CAD build for the part. Positions are in the model's coordinates, mm. A direction names the side the tool comes from. Round coordinates to 2 decimals unless told otherwise and drop trailing zeros. Write each loop counter-clockwise with the first axis right and the second up, starting at its lowest first coordinate (ties: lowest second). Pieces come first, ordered by that corner, then holes. Notation, with made-up numbers: (30.25, 4.5) - (75.25, 4.5) arc R12 cw to (75.25, 18.5) - close; hole circle Ø6 at (32.25, 32.25). An arc over 180 degrees is marked (long way). Use one line per item in the form item = value. Start each with the question number.
Item 1: Band-saw the part on A-A, the plane z = -34. List the corners of the cut face in (x, y), and give its area (3 significant figures).
Item 2: Pull direction Z, two halves, no side cores. Call faces 4 (the flat face through (-5, -3, -30.162)), 5 (the flat face through (-21, -3, -23.019)), 6 (the flat face through (52, -3, -34.925)), 7 (the flat face through (-1, -6.35, -27)): +Z half, -Z half, draft (parallel to the pull), parting line (faces both ways), or undercut.
Item 3: Drill centre lines: L1, parallel to X at y = -1.5, z = -34.5; L2, parallel to X at y = -2.75, z = -34; L3, parallel to Z at x = -41, y = -5.5. Where is each one in solid material? Low to high.
Item 4: Band-saw the part on D-D, the plane x = 43. List the corners of the cut face in (y, z), and give its area (3 significant figures).
Item 5: Band-saw the part on B-B, the plane y = -2.25. Give the number of separate pieces and of enclosed holes in the cut face, and give its area (3 significant figures).
Item 6: Band-saw the part on C-C, the plane z = -42.25. List the corners of the cut face in (x, y), and give its area (3 significant figures).
Item 7: Pin check, flat tips, straight feed: pin 1 (1.5 mm diameter, centred on y = -1, z = -39, fed in from +X); pin 2 (10 mm diameter, centred on x = 9, z = -40.5, fed in from -Y); pin 3 (1.7 mm diameter, centred on y = -3, z = -26.5, fed in from -X); pin 4 (2 mm diameter, centred on y = -3.5, z = -27.5, fed in from +X). Stop position of each tip, or through.
Item 8: Tool access for faces 1 (the flat face through (14.6, -3.13, -24.03)), 2 (the flat face through (-52, -3, -34.925)), 3 (the flat face through (47.644, -3, -33)): list every direction of +Z, -Z, +X, -X, +Y, -Y with a clear straight run to the whole face (end or side of a thin tool).
from build123d import *

# Parameters (mm, degrees)
F0_W     = 6.35
F0_H     = 9.525
F0_W_2   = 1.5875
F0_H_2   = 3.96875
F0_H_3   = 3.175
F1_DEPTH = 6.35


# Not quite as in the source:
# - a length typed as a fraction of an inch, garbled in the dataset ("3 / 203.2 mm" for 3/8 in), is restored


with BuildPart() as f1:
    # F0 (on Front) → F1 (new body)
    with BuildSketch(Plane.XZ):
        Polygon((52.4060167908, -29.36875), (55.5810167908, -23.8125), (49.2310167908, -23.8125), (49.2310167908, -20.6375), (-49.1939832092, -20.6375), (-49.1939832092, -23.8125), (-55.5439832092, -23.8125), (-52.3689832092, -29.36875), (-55.5439832092, -34.925), (-47.6064832092, -34.925), (-47.6064832092, -31.75), (-3.1564832092, -31.75), (3.1935167908, -31.75), (47.6435167908, -31.75), (47.6435167908, -34.925), (55.5810167908, -34.925), align=None)
        with BuildLine():
            Line((-36.909375, -22.225), (36.909375, -22.225))
            Line((36.909375, -22.225), (36.909375, -30.1625))
            Line((36.909375, -30.1625), (34.7265625, -30.1625))
            Line((34.7265625, -30.1625), (31.5515625, -30.1625))
            Line((31.5515625, -30.1625), (28.3765625, -30.1625))
            Line((28.3765625, -30.1625), (27.1859375, -30.1625))
            Line((27.1859375, -30.1625), (20.8359375, -30.1625))
            Line((20.8359375, -30.1625), (19.6453125, -30.1625))
            Line((19.6453125, -30.1625), (17.2640625, -30.1625))
            Line((17.2640625, -30.1625), (13.6921875, -30.1625))
            Line((13.6921875, -30.1625), (11.3109375, -30.1625))
            Line((11.3109375, -30.1625), (10.1203125, -30.1625))
            Line((10.1203125, -30.1625), (7.7390625, -30.1625))
            Line((7.7390625, -30.1625), (6.1515625, -30.1625))
            Line((6.1515625, -30.1625), (3.7703125, -30.1625))
            Line((3.7703125, -30.1625), (2.5796875, -30.1625))
            Line((2.5796875, -30.1625), (0.1984375, -30.1625))
            Line((0.1984375, -30.1625), (-1.3890625, -30.1625))
            Line((-1.3890625, -30.1625), (-3.7703125, -30.1625))
            Line((-3.7703125, -30.1625), (-4.9609375, -30.1625))
            Line((-4.9609375, -30.1625), (-6.8241157772, -30.1625))
            add(Edge.make_bspline(
                [(-8.1359375, -30.1873046875), (-7.6862010464, -30.1873046875), (-7.2364645928, -30.1795465798), (-6.8241157772, -30.1625)],
                knots=[0.5, 0.5, 0.5, 0.5, 0.5965188889, 0.5965188889, 0.5965188889, 0.5965188889], degree=3))
            add(Edge.make_bspline(
                [(-9.4477592243, -30.1625), (-9.0354104083, -30.1795465799), (-8.5856739541, -30.1873046875), (-8.1359375, -30.1873046875)],
                knots=[0.403481111, 0.403481111, 0.403481111, 0.403481111, 0.5, 0.5, 0.5, 0.5], degree=3))
            Line((-9.4477592243, -30.1625), (-11.3109375, -30.1625))
            Line((-11.3109375, -30.1625), (-12.5015625, -30.1625))
            Line((-12.5015625, -30.1625), (-14.8828125, -30.1625))
            Line((-14.8828125, -30.1625), (-16.4703125, -30.1625))
            Line((-16.4703125, -30.1625), (-18.8515625, -30.1625))
            Line((-18.8515625, -30.1625), (-20.0421875, -30.1625))
            Line((-20.0421875, -30.1625), (-22.4234375, -30.1625))
            Line((-22.4234375, -30.1625), (-24.8046875, -30.1625))
            Line((-24.8046875, -30.1625), (-27.1859375, -30.1625))
            Line((-27.1859375, -30.1625), (-28.3765625, -30.1625))
            Line((-28.3765625, -30.1625), (-30.8380988479, -30.1625))
            add(Edge.make_bspline(
                [(-31.5515625, -30.1873046875), (-31.3115619086, -30.1873046875), (-31.0715613172, -30.1779187981), (-30.8380988479, -30.1625)],
                knots=[0.5, 0.5, 0.5, 0.5, 0.5625917967, 0.5625917967, 0.5625917967, 0.5625917967], degree=3))
            add(Edge.make_bspline(
                [(-32.2650261503, -30.1625), (-32.0315636815, -30.177918798), (-31.7915630907, -30.1873046875), (-31.5515625, -30.1873046875)],
                knots=[0.4374082034, 0.4374082034, 0.4374082034, 0.4374082034, 0.5, 0.5, 0.5, 0.5], degree=3))
            Line((-32.2650261503, -30.1625), (-34.7265625, -30.1625))
            Line((-34.7265625, -30.1625), (-36.909375, -30.1625))
            Line((-36.909375, -30.1625), (-36.909375, -22.225))
        make_face(mode=Mode.SUBTRACT)
        with Locations((0.0185167908, -39.6875)):
            Rectangle(F0_W, F0_H)
        Polygon((17.2640625, -30.1625), (19.6453125, -30.1625), (19.6453125, -23.01875), (17.2640625, -23.01875), (15.478125, -25.0092855764), (13.6921875, -23.01875), (11.3109375, -23.01875), (11.3109375, -30.1625), (13.6921875, -30.1625), (13.6921875, -26.5844644236), (15.478125, -28.575), (17.2640625, -26.5844644236), align=None)
        with BuildLine():
            Line((28.3765625, -30.1625), (31.5515625, -30.1625))
            add(Edge.make_bspline(
                [(31.5515625, -30.1625), (32.7421875004, -30.1591077376), (34.5123349703, -30.1090597393), (34.7058178423, -29.8567694785), (34.7265625, -29.765625)],
                knots=[0, 0, 0, 0, 0.5486856078, 0.7169739211, 0.7169739211, 0.7169739211, 0.7169739211], degree=3))
            Line((34.7265625, -29.765625), (34.7265625, -28.971875))
            Line((34.7265625, -28.971875), (34.7265625, -24.209375))
            add(Edge.make_bspline(
                [(32.338456939, -23.01875), (33.0698998056, -23.0207151841), (33.9016308923, -23.0447678149), (34.6240389102, -23.3694667004), (34.7265625, -23.8125000002), (34.7265625, -24.209375)],
                knots=[0.1152880959, 0.1152880959, 0.1152880959, 0.1152880959, 0.4729542068, 0.722889892, 1, 1, 1, 1], degree=3))
            Line((32.338456939, -23.01875), (31.5515625, -23.01875))
            Line((31.5515625, -23.01875), (28.3765625, -23.01875))
            Line((28.3765625, -23.01875), (28.3765625, -30.1625))
        make_face()
        with Locations((31.5515625, -26.590625)):
            Rectangle(F0_W_2, F0_H_2, mode=Mode.SUBTRACT)
        Polygon((-27.1859375, -23.01875), (-27.1859375, -30.1625), (-24.8046875, -30.1625), (-24.8046875, -26.9875), (-22.4234375, -30.1625), (-20.0421875, -30.1625), (-20.0421875, -23.01875), (-22.4234375, -23.01875), (-22.4234375, -26.19375), (-24.8046875, -23.01875), align=None)
        Polygon((0.1984375, -30.1625), (2.5796875, -30.1625), (2.5796875, -23.01875), (0.1984375, -23.01875), (0.1984375, -25.4), (-1.3890625, -25.4), (-1.3890625, -23.01875), (-3.7703125, -23.01875), (-3.7703125, -30.1625), (-1.3890625, -30.1625), (-1.3890625, -27.78125), (0.1984375, -27.78125), align=None)
        with BuildLine():
            add(Edge.make_bspline(
                [(-34.7265625, -28.971875), (-34.7265625, -29.3687499998), (-34.6194398399, -29.8515743848), (-33.9447907089, -29.9651114553), (-32.920864157, -30.119185827), (-32.2650261503, -30.1625)],
                knots=[0, 0, 0, 0, 0.139450599, 0.2615766049, 0.4374082034, 0.4374082034, 0.4374082034, 0.4374082034], degree=3))
            Line((-32.2650261503, -30.1625), (-31.5515625, -30.1625))
            Line((-31.5515625, -30.1625), (-30.8380988479, -30.1625))
            add(Edge.make_bspline(
                [(-30.8380988479, -30.1625), (-30.1822608419, -30.119185827), (-29.1583342909, -29.9651114555), (-28.4836851601, -29.851574384), (-28.3765625, -29.3687500019), (-28.3765625, -28.971875)],
                knots=[0.5625917967, 0.5625917967, 0.5625917967, 0.5625917967, 0.7384233951, 0.860549401, 1, 1, 1, 1], degree=3))
            Line((-28.3765625, -28.971875), (-28.3765625, -23.01875))
            Line((-28.3765625, -23.01875), (-30.7578125, -23.01875))
            Line((-30.7578125, -23.01875), (-30.7578125, -28.575))
            Line((-30.7578125, -28.575), (-32.3453125, -28.575))
            Line((-32.3453125, -28.575), (-32.3453125, -23.01875))
            Line((-32.3453125, -23.01875), (-34.7265625, -23.01875))
            Line((-34.7265625, -23.01875), (-34.7265625, -28.971875))
        make_face()
        with BuildLine():
            add(Edge.make_bspline(
                [(-11.3109375, -29.765625), (-11.2890563147, -29.8564083098), (-11.1398834343, -30.0383555662), (-10.2076153949, -30.1310873988), (-9.4477592243, -30.1625)],
                knots=[0.1414902381, 0.1414902381, 0.1414902381, 0.1414902381, 0.2256208371, 0.403481111, 0.403481111, 0.403481111, 0.403481111], degree=3))
            Line((-9.4477592243, -30.1625), (-8.1359375, -30.1625))
            Line((-8.1359375, -30.1625), (-6.8241157772, -30.1625))
            add(Edge.make_bspline(
                [(-6.8241157772, -30.1625), (-6.0642596059, -30.1310873988), (-5.1319915657, -30.0383555662), (-4.9828186853, -29.8564083099), (-4.9609375, -29.765625)],
                knots=[0.5965188889, 0.5965188889, 0.5965188889, 0.5965188889, 0.7743791629, 0.8585097619, 0.8585097619, 0.8585097619, 0.8585097619], degree=3))
            Line((-4.9609375, -29.765625), (-4.9609375, -28.971875))
            Line((-4.9609375, -28.971875), (-4.9609375, -26.19375))
            Line((-4.9609375, -26.19375), (-8.9296875, -26.19375))
            Line((-8.9296875, -26.19375), (-8.9296875, -24.60625))
            Line((-8.9296875, -24.60625), (-7.3421875, -24.60625))
            Line((-7.3421875, -24.60625), (-7.3421875, -25.4))
            Line((-7.3421875, -25.4), (-4.9609375, -25.4))
            Line((-4.9609375, -25.4), (-4.9609375, -24.209375))
            add(Edge.make_bspline(
                [(-8.1359375, -23.01875), (-7.2216783904, -23.0187499999), (-5.8389001857, -23.1942073937), (-5.0681026979, -23.3310171279), (-4.9609375, -23.8124999986), (-4.9609375, -24.209375)],
                knots=[0.5, 0.5, 0.5, 0.5, 0.738366324, 0.8605189755, 1, 1, 1, 1], degree=3))
            add(Edge.make_bspline(
                [(-11.3109375, -24.209375), (-11.3109375, -23.8125000002), (-11.2037723021, -23.3310171272), (-10.4329748143, -23.194207394), (-9.0501966096, -23.0187500001), (-8.1359375, -23.01875)],
                knots=[0, 0, 0, 0, 0.1394810245, 0.261633676, 0.5, 0.5, 0.5, 0.5], degree=3))
            Line((-11.3109375, -24.209375), (-11.3109375, -26.9875))
            Line((-11.3109375, -26.9875), (-7.3421875, -26.9875))
            Line((-7.3421875, -26.9875), (-7.3421875, -28.575))
            Line((-7.3421875, -28.575), (-8.9296875, -28.575))
            Line((-8.9296875, -28.575), (-8.9296875, -27.78125))
            Line((-8.9296875, -27.78125), (-11.3109375, -27.78125))
            Line((-11.3109375, -27.78125), (-11.3109375, -28.971875))
            Line((-11.3109375, -28.971875), (-11.3109375, -29.765625))
        make_face()
        Polygon((20.8359375, -30.1625), (27.1859375, -30.1625), (27.1859375, -28.575), (23.2171875, -28.575), (23.2171875, -27.384375), (26.3921875, -27.384375), (26.3921875, -25.796875), (23.2171875, -25.796875), (23.2171875, -24.60625), (27.1859375, -24.60625), (27.1859375, -23.01875), (20.8359375, -23.01875), align=None)
        Polygon((-16.8671875, -23.01875), (-18.8515625, -30.1625), (-16.4703125, -30.1625), (-16.0734375, -28.73375), (-15.2796875, -28.73375), (-14.8828125, -30.1625), (-12.5015625, -30.1625), (-14.4859375, -23.01875), align=None)
        Polygon((-16.160156063, -27.14625), (-15.6765625, -25.4053131732), (-15.192968937, -27.14625), align=None, mode=Mode.SUBTRACT)
        Polygon((7.7390625, -30.1625), (10.1203125, -30.1625), (8.1359375, -23.01875), (5.7546875, -23.01875), (3.7703125, -30.1625), (6.1515625, -30.1625), (6.5484375, -28.73375), (7.3421875, -28.73375), align=None)
        Polygon((6.461718937, -27.14625), (6.9453125, -25.4053131732), (7.428906063, -27.14625), align=None, mode=Mode.SUBTRACT)
        with Locations((0.0185167908, -33.3375)):
            Rectangle(F0_W, F0_H_3)
        with BuildLine():
            Line((-8.1359375, -30.1625), (-9.4477592243, -30.1625))
            add(Edge.make_bspline(
                [(-9.4477592243, -30.1625), (-9.0354104083, -30.1795465799), (-8.5856739541, -30.1873046875), (-8.1359375, -30.1873046875)],
                knots=[0.403481111, 0.403481111, 0.403481111, 0.403481111, 0.5, 0.5, 0.5, 0.5], degree=3))
            Line((-8.1359375, -30.1873046875), (-8.1359375, -30.1625))
        make_face()
        with BuildLine():
            Line((-6.8241157772, -30.1625), (-8.1359375, -30.1625))
            Line((-8.1359375, -30.1625), (-8.1359375, -30.1873046875))
            add(Edge.make_bspline(
                [(-8.1359375, -30.1873046875), (-7.6862010464, -30.1873046875), (-7.2364645928, -30.1795465798), (-6.8241157772, -30.1625)],
                knots=[0.5, 0.5, 0.5, 0.5, 0.5965188889, 0.5965188889, 0.5965188889, 0.5965188889], degree=3))
        make_face()
        with BuildLine():
            Line((-31.5515625, -30.1625), (-32.2650261503, -30.1625))
            add(Edge.make_bspline(
                [(-32.2650261503, -30.1625), (-32.0315636815, -30.177918798), (-31.7915630907, -30.1873046875), (-31.5515625, -30.1873046875)],
                knots=[0.4374082034, 0.4374082034, 0.4374082034, 0.4374082034, 0.5, 0.5, 0.5, 0.5], degree=3))
            Line((-31.5515625, -30.1873046875), (-31.5515625, -30.1625))
        make_face()
        with BuildLine():
            Line((-30.8380988479, -30.1625), (-31.5515625, -30.1625))
            Line((-31.5515625, -30.1625), (-31.5515625, -30.1873046875))
            add(Edge.make_bspline(
                [(-31.5515625, -30.1873046875), (-31.3115619086, -30.1873046875), (-31.0715613172, -30.1779187981), (-30.8380988479, -30.1625)],
                knots=[0.5, 0.5, 0.5, 0.5, 0.5625917967, 0.5625917967, 0.5625917967, 0.5625917967], degree=3))
        make_face()
    extrude(amount=F1_DEPTH)


solid = f1.part
Determined:
q1.outline = (-55.02, -6.35) - (-47.61, -6.35) - (-47.61, 0) - (-55.02, 0) - close; (-3.16, -6.35) - (3.19, -6.35) - (3.19, 0) - (-3.16, 0) - close; (47.64, -6.35) - (55.05, -6.35) - (55.05, 0) - (47.64, 0) - close
q1.area = 134 mm²
q2.face_4 = undercut
q2.face_5 = undercut
q2.face_6 = -Z half
q2.face_7 = draft
q3.L1 = -55.3 to -47.61, -3.16 to 3.19, 47.64 to 55.34
q3.L2 = -55.02 to -47.61, -3.16 to 3.19, 47.64 to 55.05
q3.L3 = -31.75 to -20.64
q4.outline = (-6.35, -31.75) - (0, -31.75) - (0, -20.64) - (-6.35, -20.64) - close
q4.area = 70.6 mm²
q5.separate_pieces = 1
q5.enclosed_holes = 9
q5.area = 1,030 mm²
q6.outline = (-3.16, -6.35) - (3.19, -6.35) - (3.19, 0) - (-3.16, 0) - close
q6.area = 40.3 mm²
q7.pin_1 = 3.19
q7.pin_2 = through
q7.pin_3 = -54.49
q7.pin_4 = 54.05
q8.face_1 = +Y, -Y
q8.face_2 = -Z, -X, +Y, -Y
q8.face_3 = -Z, +Y, -Y
